Autodesk Inventor part; units mm, degrees
ref_plane "YZ Plane" through (0, 0, 0) normal (1, 0, 0) x (0, 1, 0)
ref_plane "XZ Plane" through (0, 0, 0) normal (0, 1, 0) x (-1, 0, 0)
ref_plane "XY Plane" through (0, 0, 0) normal (0, 0, 1) x (1, 0, 0)
sketch "Sketch1" plane through (0, 0, 0) normal (0, 0, 1) x (1, 0, 0)
  line L0 (0, 0) -> (10, 0)
  line L1 (10, 0) -> (10, 3)
  line L2 (10, 3) -> (0, 3)
  line L3 (0, 3) -> (0, 0)
  line L4 (30, 0) -> (40, 0)
  line L5 (40, 0) -> (40, 3)
  line L6 (40, 3) -> (30, 3)
  line L7 (30, 3) -> (30, 0)
  line L8 (0, 0) -> (40, 0)
  line L9 (40, 0) -> (40, 40)
  line L10 (40, 40) -> (0, 40)
  line L11 (0, 40) -> (0, 0)
  circle A0 centre (20, -31) radius 7.5
  circle A1 centre (20, -31) radius 20
  line L12 (-4, 44) -> (44, 44)
  line L13 (44, 44) -> (44, 0)
  line L14 (44, 0) -> (-4, 0)
  line L15 (-4, 0) -> (-4, 44)
  line L16 (-4, 0) -> (0.1522, -33.4628)
  line L17 (44, 0) -> (39.8478, -33.4628)
  circle A2 centre (20, 28) radius 4.25
  line L18 (10, 3) -> (30, 3)
  point P0 (20, 0)
  point P1 (1.3083, -38.1147)
  point P2 (38.6917, -38.1147)
  point P3 (30, 1.3205)
  point P4 (10, 1.3205)
  point P5 (8, 0)
  point P6 (32, 0)
  dimension "d0" = 10
  dimension "d1" = 3
  dimension "d2" = 10
  dimension "d3" = 20
  dimension "d4" = 40
  dimension "d5" = 15
  dimension "d6" = 40
  dimension "d7" = 31
  dimension "d9" = 4
  dimension "d10" = 4
  dimension "d11" = 4
  dimension "d12" = 8.5
  dimension "d17" = 25
extrude "Plate1" add sketch "Sketch1" along normal blind 3 contours L14 L15 L12 L13 L5 L9 L10 L11 L3 | L0 L8 L4 L14 L17 A1 L16 | L1 L18 L7 L8 | L11 L10 L9 L6 L18 L2 | A1
chamfer "Corner Chamfer1" distance 6 angle 45 2 edges at (-4, 44, 1.5) (44, 44, 1.5)
equation "\"d10\" = d9"
equation "\"d11\" = d10"
equation "\"d8\" = Thickness"
equation "\"BendRadius\" = Thickness"
equation "\"BendReliefWidth\" = Thickness"
equation "\"BendReliefDepth\" = 0.5 * Thickness"
equation "\"CornerReliefSize\" = 4 * Thickness"
equation "\"MinimumRemnant\" = 2 * Thickness"
equation "\"TransitionRadius\" = BendRadius"
equation "\"JacobiRadiusSize\" = BendRadius"
equation "\"GapSize\" = Thickness"
properties part number "A_beam_end_mound_2"
Part model, mm, in its own coordinate system. A direction names the side the tool comes from. Round coordinates to 2 decimals unless told otherwise and drop trailing zeros. Order: outer loops, then holes, each group sorted by start corner. A loop starts at its lowest first (then second) coordinate and runs counter-clockwise, first axis right, second up. Notation, with made-up numbers: M -3,-6.75 L 8,-6.75 A29 ccw 8,13.25 Z; hole C 63,30.5 d4. An arc over 180 degrees is marked long. Put each result on its own line as item: value. Start each with the question number.
1. Drill centre lines: probe 1 along Y at (x, z) = (20, 2.3); probe 2 along Y at (x, z) = (19, 1.7); probe 3 along Y at (x, z) = (24.5, 0.75). Where is each one in solid material? Low to high. Write a range as [from, to].
2. Slice it at D-D on y = -26.5. List the corners of the cut face in (x, z), then the cut area to 3 significant figures.
3. Slice it at A-A on x = 20. List the corners of the cut face in (y, z).
4. Tool access for faces 1 (the face through (30, 2, 1)), 2 (the face through (41, 41, 1)): list every direction of +Z, -Z, +X, -X, +Y, -Y with a clear straight run to the whole face (end or side of a thin tool).
5. Slice it at C-C on x = 34. List the corners of the cut face in (y, z).
6. Two-plate mould, pull along Y, no slides. Class faces 3 (the face through (5, 0, 1)), 4 (the face through (-4, 19, 1)), 5 (the face through (-1.953, -16.497, 1.479)): +Y half, -Y half, draft (parallel to the pull), parting line (faces both ways), or undercut.
7. Slice it at B-B on y = 2. List the corners of the cut face in (x, z), then the cut area to 3 significant figures.
8. Drop flat-ended pins along their axis: pin 1 (0.9 mm diameter, centred on x = 6, z = 1, fed in from -Y); pin 2 (12 mm diameter, centred on x = 9, y = 25.5, fed in from -Z). Give the stop position or say it passes through.
Findings:
1. probe 1: [-51, -38.5], [-23.5, 23.75], [32.25, 44]
1. probe 2: [-50.97, -38.43], [-23.57, 23.87], [32.13, 44]
1. probe 3: [-50.49, -37], [-25, 44]
2. outline: M -0.71,0 L 14,0 L 14,3 L -0.71,3 Z; M 26,0 L 40.71,0 L 40.71,3 L 26,3 Z
2. area: 88.3 mm2
3. outline: M -51,0 L -38.5,0 L -38.5,3 L -51,3 Z; M -23.5,0 L 23.75,0 L 23.75,3 L -23.5,3 Z; M 32.25,0 L 44,0 L 44,3 L 32.25,3 Z
4. face 1: +Z, -Z
4. face 2: +Z, -Z, +X, +Y
5. outline: M -45.28,0 L 0,0 L 0,3 L -45.28,3 Z; M 3,0 L 44,0 L 44,3 L 3,3 Z
6. face 3: undercut
6. face 4: draft
6. face 5: -Y half
7. outline: M -4,0 L 0,0 L 0,3 L -4,3 Z; M 10,0 L 30,0 L 30,3 L 10,3 Z; M 40,0 L 44,0 L 44,3 L 40,3 Z
7. area: 84.0 mm2
8. pin 1: y = -45.71
8. pin 2: z = 0
